Part print with two shaded views. Sizes in mm from the minimum x, y, z corner. A direction names the side the tool comes from. Round coordinates to 2 decimals unless told otherwise and drop trailing zeros. Loops run counter-clockwise (first coordinate to the right, second up) from the corner with the lowest first, then second, coordinate; pieces in that order, holes last. Notation, with made-up numbers: (26, 10) -> (64, 10) arc R25 ccw to (64, 35) -> close; hole circle Ø5 at (46.25, -10.5). An arc over 180 degrees is marked (long way). Use a Markdown table: item, result. Add a question column.
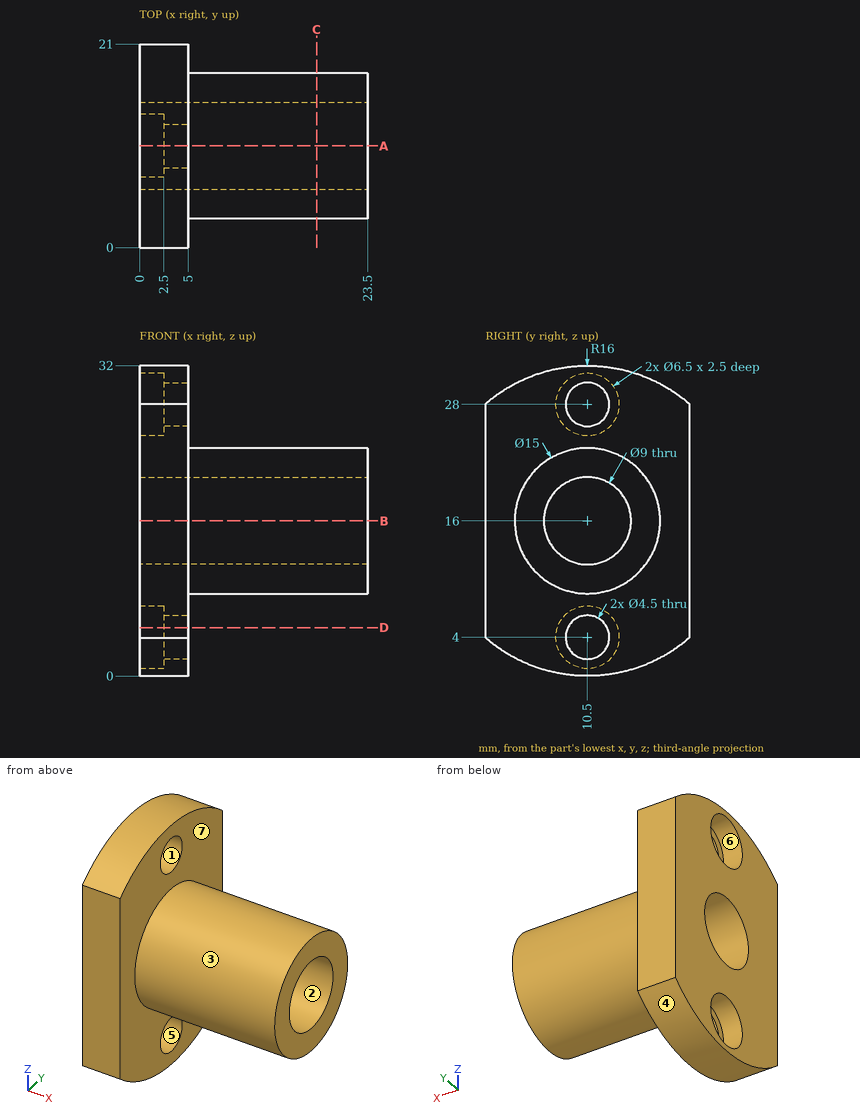
1) Pin check, flat tips, straight feed: pin 1 Ø11.5 at (y, z) = (10.5, 16) entering from +X; pin 2 Ø6 at (y, z) = (10.5, 28) entering from +X; pin 3 Ø2 at (y, z) = (12, 5) entering from -X; pin 4 Ø8 at (x, z) = (16.5, 26.5) entering from +Y. Stop position of each tip, or through.
2) Cut at C-C on x = 18.25. Write the cut outline in (y, z), and give its area (3 significant figures).
3) Tool access for the marked faces 5, 6 and 7: list every direction of +Z, -Z, +X, -X, +Y, -Y with a clear straight run to the whole face (end or side of a thin tool).
4) Cut at D-D on z = 5. Write the cut outline in (x, y).
5) Cut at A-A on y = 10.5. Write the cut outline in (x, z).
6) Wall check: probe 1 along Y at (x, z) = (3.6, 4); probe 2 along Y at (x, z) = (5.5, 16); probe 3 along X at (y, z) = (3, 14). Give the ranges that are in metal, low to high. Write a range as from..to.
7) Cut at B-B on z = 16. Write the cut outline in (x, y).
8) Pull direction Z, two halves, no side cores. Call the marked faces 1, 2, 3 and 4: +Z half, -Z half, draft (parallel to the pull), parting line (faces both ways), or undercut.
Established:
| question | item | result |
|---|---|---|
| 1 | pin 1 | stops at x = 23.5 |
| 1 | pin 2 | stops at x = 5 |
| 1 | pin 3 | stops at x = 2.5 |
| 1 | pin 4 | stops at y = 14.24 |
| 2 | outline | circle Ø15 at (10.5, 16); hole circle Ø9 at (10.5, 16) |
| 2 | area | 113 mm^2 |
| 3 | face 5 | +X, -X |
| 3 | face 6 | -X |
| 3 | face 7 | +X |
| 4 | outline | (0, 0) -> (5, 0) -> (5, 8.48) -> (2.5, 8.48) -> (2.5, 7.41) -> (0, 7.41) -> close; (0, 13.59) -> (2.5, 13.59) -> (2.5, 12.52) -> (5, 12.52) -> (5, 21) -> (0, 21) -> close |
| 5 | outline | (0, 0) -> (5, 0) -> (5, 1.75) -> (2.5, 1.75) -> (2.5, 0.75) -> (0, 0.75) -> close; (0, 7.25) -> (2.5, 7.25) -> (2.5, 6.25) -> (5, 6.25) -> (5, 8.5) -> (23.5, 8.5) -> (23.5, 11.5) -> (0, 11.5) -> close; (0, 20.5) -> (23.5, 20.5) -> (23.5, 23.5) -> (5, 23.5) -> (5, 25.75) -> (2.5, 25.75) -> (2.5, 24.75) -> (0, 24.75) -> close; (0, 31.25) -> (2.5, 31.25) -> (2.5, 30.25) -> (5, 30.25) -> (5, 32) -> (0, 32) -> close |
| 6 | probe 1 | y = 0..8.25, 12.75..21 |
| 6 | probe 2 | y = 3..6, 15..18 |
| 6 | probe 3 | x = 0..5 |
| 7 | outline | (0, 0) -> (5, 0) -> (5, 3) -> (23.5, 3) -> (23.5, 6) -> (0, 6) -> close; (0, 15) -> (23.5, 15) -> (23.5, 18) -> (5, 18) -> (5, 21) -> (0, 21) -> close |
| 8 | face 1 | undercut |
| 8 | face 2 | undercut |
| 8 | face 3 | parting line |
| 8 | face 4 | -Z half |
